from build123d import *

# Parameters (mm, degrees)
F0_R     = 1.4986
F0_W     = 10.0076
F0_H     = 30.988
F1_DEPTH = 4.7625
F2_R     = 3.9878
F4_DEPTH = 25.4
F5_R     = 6.35
F6_R     = 12.7


with BuildPart() as f1:
    # F0 (on Top) → F1 (new body)
    with BuildSketch(Plane.XY):
        with BuildLine():
            Line((104.4956, 113.6142), (-104.4956, 113.6142))
            ThreePointArc((-104.4956, 113.6142), (-110.943424, 110.943424), (-113.6142, 104.4956))
            Line((-113.6142, 104.4956), (-113.6142, -104.4956))
            ThreePointArc((-113.6142, -104.4956), (-110.943424, -110.943424), (-104.4956, -113.6142))
            Line((-104.4956, -113.6142), (104.4956, -113.6142))
            ThreePointArc((104.4956, -113.6142), (110.943424, -110.943424), (113.6142, -104.4956))
            Line((113.6142, -104.4956), (113.6142, 104.4956))
            ThreePointArc((113.6142, 104.4956), (110.943424, 110.943424), (104.4956, 113.6142))
        make_face()
        with Locations((-104.4956, -104.4956)):
            Circle(F0_R, mode=Mode.SUBTRACT)
        with Locations((-93.4974, -35.0012)):
            Circle(F0_R, mode=Mode.SUBTRACT)
        with Locations((-85.0011, -35.0012)):
            Rectangle(F0_W, F0_H, mode=Mode.SUBTRACT)
        with Locations((-76.5048, -35.0012)):
            Circle(F0_R, mode=Mode.SUBTRACT)
        with Locations((104.4956, -104.4956)):
            Circle(F0_R, mode=Mode.SUBTRACT)
        with Locations((0, -21.9964)):
            Circle(F0_R, mode=Mode.SUBTRACT)
        with Locations((-93.4974, 35.0012)):
            Circle(F0_R, mode=Mode.SUBTRACT)
        with Locations((-85.0011, 35.0012)):
            Rectangle(F0_W, F0_H, mode=Mode.SUBTRACT)
        with Locations((-76.5048, 35.0012)):
            Circle(F0_R, mode=Mode.SUBTRACT)
        with Locations((-104.4956, 104.4956)):
            Circle(F0_R, mode=Mode.SUBTRACT)
        with Locations((0, 21.9964)):
            Circle(F0_R, mode=Mode.SUBTRACT)
        with Locations((75.0062, 0)):
            Circle(F0_R, mode=Mode.SUBTRACT)
        with Locations((85.0011, 0)):
            Rectangle(F0_W, F0_H, mode=Mode.SUBTRACT)
        with Locations((94.996, 0)):
            Circle(F0_R, mode=Mode.SUBTRACT)
        with Locations((104.4956, 104.4956)):
            Circle(F0_R, mode=Mode.SUBTRACT)
    extrude(amount=F1_DEPTH)

    # F2
    f2_edges = [f1.edges().sort_by_distance(p)[0] for p in [
        (-79.9973, 50.4952, 2.38125),
        (-79.9973, -19.5072, 2.38125),
        (90.0049, 15.494, 2.38125),
        (79.9973, 15.494, 2.38125),
        (-90.0049, 50.4952, 2.38125),
        (-90.0049, -19.5072, 2.38125),
        (79.9973, -15.494, 2.38125),
        (-90.0049, -50.4952, 2.38125),
        (-90.0049, 19.5072, 2.38125),
        (-79.9973, -50.4952, 2.38125),
        (-79.9973, 19.5072, 2.38125),
        (90.0049, -15.494, 2.38125),
    ]]
    fillet(f2_edges, radius=F2_R)


with BuildPart() as f4:
    # F3 (on Top) → F4 (new body)
    with BuildSketch(Plane.XY):
        with BuildLine():
            Line((-98.494212, 51.695601), (-103.676097, 39.23368))
            ThreePointArc((-103.676097, 39.23368), (-104.521, 35.0012), (-103.676097, 30.76872))
            Line((-103.676097, 30.76872), (-98.494212, 18.306799))
            ThreePointArc((-98.494212, 18.306799), (-94.839742, 0), (-98.494212, -18.306799))
            Line((-98.494212, -18.306799), (-103.676097, -30.76872))
            ThreePointArc((-103.676097, -30.76872), (-104.521, -35.0012), (-103.676097, -39.23368))
            Line((-103.676097, -39.23368), (-98.494212, -51.695601))
            ThreePointArc((-98.494212, -51.695601), (-97.609151, -53.451471), (-96.478631, -55.060303))
            Line((-96.478631, -55.060303), (-107.133793, -95.76698))
            ThreePointArc((-107.133793, -95.76698), (-109.57774, -112.066644), (-95.418055, -103.631288))
            Line((-95.418055, -103.631288), (-7.629691, -37.659037))
            ThreePointArc((-7.629691, -37.659037), (0, -35.111761), (7.629691, -37.659037))
            Line((7.629691, -37.659037), (95.418055, -103.631288))
            ThreePointArc((95.418055, -103.631288), (109.233289, -112.286824), (107.904862, -96.038308))
            Line((107.904862, -96.038308), (95.352953, -21.275418))
            ThreePointArc((95.352953, -21.275418), (96.777145, -19.680378), (97.93189, -17.880645))
            Line((97.93189, -17.880645), (104.71596, -5.200205))
            ThreePointArc((104.71596, -5.200205), (106.0196, 0), (104.71596, 5.200205))
            Line((104.71596, 5.200205), (97.93189, 17.880645))
            ThreePointArc((97.93189, 17.880645), (96.777145, 19.680378), (95.352953, 21.275418))
            Line((95.352953, 21.275418), (107.904862, 96.038308))
            ThreePointArc((107.904862, 96.038308), (109.233289, 112.286824), (95.418055, 103.631288))
            Line((95.418055, 103.631288), (7.629691, 37.659037))
            ThreePointArc((7.629691, 37.659037), (0, 35.111761), (-7.629691, 37.659037))
            Line((-7.629691, 37.659037), (-95.418055, 103.631288))
            ThreePointArc((-95.418055, 103.631288), (-109.57774, 112.066644), (-107.133793, 95.76698))
            Line((-107.133793, 95.76698), (-96.478631, 55.060303))
            ThreePointArc((-96.478631, 55.060303), (-97.609151, 53.451471), (-98.494212, 51.695601))
        make_face()
        with BuildLine():
            Line((-93.884154, -89.512986), (-83.387341, -61.096307))
            ThreePointArc((-83.387341, -61.096307), (-80.919825, -59.955425), (-78.444317, -58.831989))
            ThreePointArc((-78.444317, -58.831989), (-58.568879, -50.556323), (-38.262066, -43.404188))
            Line((-38.262066, -43.404188), (-93.884154, -89.512986))
        make_face(mode=Mode.SUBTRACT)
        with BuildLine():
            Line((-71.507988, 18.306799), (-66.326103, 30.76872))
            ThreePointArc((-66.326103, 30.76872), (-66.055449, 31.489672), (-65.835789, 32.227761))
            ThreePointArc((-65.835789, 32.227761), (-62.636313, 36.255281), (-57.503646, 36.591882))
            ThreePointArc((-57.503646, 36.591882), (-36.852243, 29.653537), (-15.852003, 23.856035))
            ThreePointArc((-15.852003, 23.856035), (-12.374368, 21.606411), (-11.0236, 17.691033))
            Line((-11.0236, 17.691033), (-11.0236, -17.691033))
            ThreePointArc((-11.0236, -17.691033), (-12.374368, -21.606411), (-15.852003, -23.856035))
            ThreePointArc((-15.852003, -23.856035), (-36.852243, -29.653537), (-57.503646, -36.591882))
            ThreePointArc((-57.503646, -36.591882), (-62.636313, -36.255281), (-65.835789, -32.227761))
            ThreePointArc((-65.835789, -32.227761), (-66.055449, -31.489672), (-66.326103, -30.76872))
            Line((-66.326103, -30.76872), (-71.507988, -18.306799))
            ThreePointArc((-71.507988, -18.306799), (-75.162458, 0), (-71.507988, 18.306799))
        make_face(mode=Mode.SUBTRACT)
        with BuildLine():
            ThreePointArc((21.342663, -29.378585), (51.05322, -26.015895), (80.935105, -24.968148))
            Line((80.935105, -24.968148), (96.6187, -91.779831))
            Line((96.6187, -91.779831), (21.342663, -29.378585))
        make_face(mode=Mode.SUBTRACT)
        with BuildLine():
            ThreePointArc((59.194505, 12.782899), (64.216841, 9.867757), (64.768196, 4.086934))
            ThreePointArc((64.768196, 4.086934), (63.9826, 0), (64.768196, -4.086934))
            ThreePointArc((64.768196, -4.086934), (64.216841, -9.867757), (59.194505, -12.782899))
            ThreePointArc((59.194505, -12.782899), (38.717595, -14.359129), (18.349308, -16.989965))
            ThreePointArc((18.349308, -16.989965), (13.242816, -15.538146), (11.0236, -10.715374))
            Line((11.0236, -10.715374), (11.0236, 10.715374))
            ThreePointArc((11.0236, 10.715374), (13.242816, 15.538146), (18.349308, 16.989965))
            ThreePointArc((18.349308, 16.989965), (38.717595, 14.359129), (59.194505, 12.782899))
        make_face(mode=Mode.SUBTRACT)
        with BuildLine():
            ThreePointArc((-38.262066, 43.404188), (-61.103294, 51.539678), (-83.387341, 61.096307))
            Line((-83.387341, 61.096307), (-93.884154, 89.512986))
            Line((-93.884154, 89.512986), (-38.262066, 43.404188))
        make_face(mode=Mode.SUBTRACT)
        with BuildLine():
            ThreePointArc((80.935105, 24.968148), (51.05322, 26.015895), (21.342663, 29.378585))
            Line((21.342663, 29.378585), (96.6187, 91.779831))
            Line((96.6187, 91.779831), (80.935105, 24.968148))
        make_face(mode=Mode.SUBTRACT)
    extrude(amount=F4_DEPTH)

    # F5
    f5_edges = [f4.edges().sort_by_distance(p)[0] for p in [
        (80.935105, -24.968148, 12.7),
        (96.6187, 91.779831, 12.7),
        (-93.884154, 89.512986, 12.7),
        (-83.387341, -61.096307, 12.7),
        (21.342663, -29.378585, 12.7),
        (96.6187, -91.779831, 12.7),
        (-93.884154, -89.512986, 12.7),
        (-38.262066, -43.404188, 12.7),
        (80.935105, 24.968148, 12.7),
        (-38.262066, 43.404188, 12.7),
        (-83.387341, 61.096307, 12.7),
        (21.342663, 29.378585, 12.7),
    ]]
    fillet(f5_edges, radius=F5_R)

    # F6
    f6_edges = [f4.edges().sort_by_distance(p)[0] for p in [
        (-95.418055, 103.631288, 12.7),
        (95.418055, 103.631288, 12.7),
        (-107.133793, -95.76698, 12.7),
        (-107.133793, 95.76698, 12.7),
        (95.418055, -103.631288, 12.7),
        (-95.418055, -103.631288, 12.7),
        (107.904862, -96.038308, 12.7),
        (107.904862, 96.038308, 12.7),
    ]]
    fillet(f6_edges, radius=F6_R)

    # F7: intersect F1
    add(f1.part, mode=Mode.INTERSECT)


solid = f4.part
The model under review builds one solid part; all positions refer to its coordinate system, in mm. A direction names the side the tool comes from. Give positions to 0.01 mm unless a question says otherwise; leave off trailing zeros. Loops run counter-clockwise (first coordinate to the right, second up) from the corner with the lowest first, then second, coordinate; pieces in that order, holes last. Notation, with made-up numbers: (-34, 80) -> (-26, 80) arc R10 cw to (-26, 86) -> close; hole circle Ø1 at (51.5, 78.5). An arc over 180 degrees is marked (long way). Answer as a JSON object with one key per item and string values. Group by question number.
Q1. Insertion check: pin 1 (1.4 mm diameter, centred on y = 38, z = 3, fed in from +X); pin 2 (1.6 mm diameter, centred on x = 85.5, z = 2, fed in from +Y); pin 3 (0.6 mm diameter, centred on x = -84.5, z = 1, fed in from +Y). Each pin has a flat end and moves straight along its axis. Give the tip position at first contact, or say it passes through.
Q2. Tool access review of faces 1 (the flat face through (101.276, -11.629, 2.348)), 2 (the flat face through (-68.953, 24.451, 2.348)), 3 (the flat face through (-101.12, 24.62, 2.35)): name each direction out of +Z, -Z, +X, -X, +Y, -Y from which nothing blocks a thin tool from reaching the whole face with its end or side.
Q3. Take a section at C-C (z = 0.85). State how many separate pieces and enclosed holes the cut face has, plus the area to 3 significant figures.
Q4. Draft analysis for pull direction X (two halves, no side actions). For faces 4 (the flat face through (-2, 2, 4.762)), 5 (the flat face through (-48.8, 68.6, 2.3)), 6 (the flat face through (101.27, -56.53, 2.35)), state which applies: pulls with the +X half, pulls with the -X half, needs draft (parallel to the pull), parting line crosses it, or undercut.
Q5. Take a section at A-A (x = 49). Write out the cut boundary in (y, z).
Q6. Take a section at B-B (x = -51). Write out the cut boundary in (y, z), plus the area to 3 significant figures.
Q7. Wall thickness on line 1 along X through (y, z) = (-40, 3.4); line 2 along X through (y, z) = (55, 3.05); line 3 along Y through (x, z) = (39.5, 4.25): over which ranges is each line inside the solid? List them lowest first.
Answer below:
{
 "1": {"pin 1": "stops at x = 98.28", "pin 2": "stops at y = 96.78", "pin 3": "stops at y = 95.65"},
 "2": {"face 1": "+Z, -Z, +X", "face 2": "+Z, -Z", "face 3": "+Z, -Z, -X"},
 "3": {"separate pieces": "1", "enclosed holes": "21", "area": "18,500 mm2"},
 "4": {"face 4": "needs draft", "face 5": "undercut", "face 6": "pulls with the +X half"},
 "5": {"outline": "(-68.75, 0) -> (-52.31, 0) -> (-52.31, 4.76) -> (-68.75, 4.76) -> close; (-26.17, 0) -> (-13.43, 0) -> (-13.43, 4.76) -> (-26.17, 4.76) -> close; (13.43, 0) -> (26.17, 0) -> (26.17, 4.76) -> (13.43, 4.76) -> close; (52.31, 0) -> (68.75, 0) -> (68.75, 4.76) -> (52.31, 4.76) -> close"},
 "6": {"outline": "(-70.25, 0) -> (-34.27, 0) -> (-34.27, 4.76) -> (-70.25, 4.76) -> close; (34.27, 0) -> (70.25, 0) -> (70.25, 4.76) -> (34.27, 4.76) -> close", "area": "343 mm2"},
 "7": {"line 1": "x = -103.36 to -90, -80 to -10.74, 10.74 to 34.16, 84.46 to 98.5", "line 2": "x = -96.53 to -30.71, 30.71 to 52.25, 87.98 to 101.01", "line 3": "y = -61.61 to -44.43, -27.05 to -14.28, 14.28 to 27.05, 44.43 to 61.61"}
}
